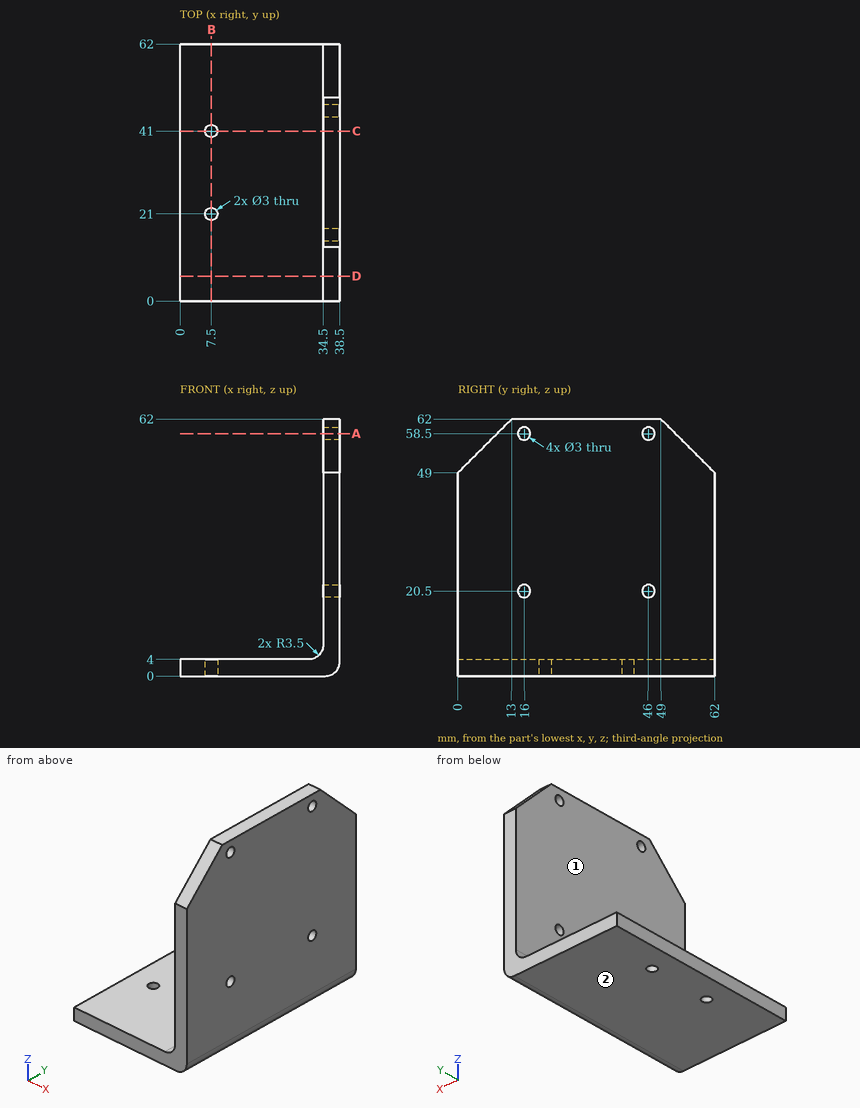
The drawing under review shows one solid part. Ordinate dimensions are in mm from its lowest x, y, z. A direction names the side the tool comes from. Round coordinates to 2 decimals unless told otherwise and drop trailing zeros. Write each loop counter-clockwise with the first axis right and the second up, starting at its lowest first coordinate (ties: lowest second). Pieces come first, ordered by that corner, then holes. Notation, with made-up numbers: M 55,-36.5 L 112,-36.5 A20 ccw 112,-26.5 Z; hole C -38.5,22.5 d1. An arc over 180 degrees is marked long. One line per item, written item: value. Start each with the question number.
(1) We need section C-C (y = 41). Give the boundary of the cut face in (x, z).
(2) We need section B-B (x = 7.5). Give the boundary of the cut face in (y, z), and give its area (3 significant figures).
(3) We need section D-D (y = 6). Give the boundary of the cut face in (x, z), and give its area (3 significant figures).
(4) Wall thickness on line 1 (Y direction, x = 7.5, z = 1.6); line 2 (X direction, y = 11, z = 18); line 3 (Z direction, x = 25, y = 57.5): over which ranges is each line inside the solid? List them lowest first.
(5) Machinability: for the marked faces 1 and 2, which of the approach directions +Z, -Z, +X, -X, +Y, -Y give a long, thin tool a straight path to every point of the face, cutting with its end or side? Answer none if there is none.
(6) Insertion check: pin 1 (5 mm diameter, centred on y = 46, z = 20.5, fed in from -X); pin 2 (10 mm diameter, centred on x = 26, z = 34.5, fed in from -Y); pin 3 (5 mm diameter, centred on x = 7.5, y = 41, fed in from +Z). Each pin has a flat end and moves straight along its axis. Give the tip position at first contact, or say it passes through.
(7) We need section A-A (z = 58.5). Give the boundary of the cut face in (x, y).
Result:
1. outline: M 0,0 L 6,0 L 6,4 L 0,4 Z; M 9,0 L 35,0 A3.5 ccw 38.5,3.5 L 38.5,62 L 34.5,62 L 34.5,7.5 A3.5 cw 31,4 L 9,4 Z
2. outline: M 0,0 L 19.5,0 L 19.5,4 L 0,4 Z; M 22.5,0 L 39.5,0 L 39.5,4 L 22.5,4 Z; M 42.5,0 L 62,0 L 62,4 L 42.5,4 Z
2. area: 224 mm²
3. outline: M 0,0 L 35,0 A3.5 ccw 38.5,3.5 L 38.5,55 L 34.5,55 L 34.5,7.5 A3.5 cw 31,4 L 0,4 Z
3. area: 358 mm²
4. line 1: 0 to 19.5, 22.5 to 39.5, 42.5 to 62
4. line 2: 34.5 to 38.5
4. line 3: 0 to 4
5. face 1: +Z, -X, +Y, -Y
5. face 2: -Z, +X, -X, +Y, -Y
6. pin 1: x = 34.5
6. pin 2: through
6. pin 3: z = 4
7. outline: M 34.5,9.5 L 38.5,9.5 L 38.5,14.5 L 34.5,14.5 Z; M 34.5,17.5 L 38.5,17.5 L 38.5,44.5 L 34.5,44.5 Z; M 34.5,47.5 L 38.5,47.5 L 38.5,52.5 L 34.5,52.5 Z
